Check sheet for the modelled part. Datum: model origin and axes. Units: mm. Face numbers are marked on the shaded views. A direction names the side the tool comes from. Round coordinates to 2 decimals unless told otherwise and drop trailing zeros. Order: outer loops, then holes, each group sorted by start corner. A loop starts at its lowest first (then second) coordinate and runs counter-clockwise, first axis right, second up. Notation, with made-up numbers: M 59,19 L 79,19 A21 cw 79,32 Z; hole C 53.5,-9.5 d4. An arc over 180 degrees is marked long. One line per item, written item: value. Start each with the question number.
(1) Cross-section at B-B, the plane y = -57.5. Enter the section's corners in (x, z), and give its area (3 significant figures).
(2) Cross-section at A-A, the plane x = -85. Enter the section's corners in (y, z).
(3) Access from +Z, -Z, +X, -X, +Y, -Y to the whole of each face (thin tool, end or side, straight path). Record for the marked faces 1 and 2.
(4) Thickness scan on L1, parallel to Z at x = -85, y = -61.7; L2, parallel to Z at x = -82.25, y = -58; L3, parallel to X at y = -64.5, z = -4. Record the ranges inside material, lowest first.
(5) Release check for a two-part mould opening along X. For the marked faces 3, 4, 5 and 6 record: released by +X, released by -X, zero draft, split by the parting line, or undercut.
(6) Cross-section at C-C, the plane y = -64.5. Enter the section's corners in (x, z).
(7) Depth check by flat-ended pin: pin 1 Ø3.5 at (x, z) = (-85.5, 8) entering from +Y; pin 2 Ø8 at (x, z) = (-85, 0) entering from -Y; pin 3 Ø1.6 at (x, z) = (-85, -19.25) entering from -Y. Enter the tip coordinate at first touch or a pass-through.
(8) Cross-section at D-D, the plane z = 8.25. Enter the section's corners in (x, y), and give its area (3 significant figures).
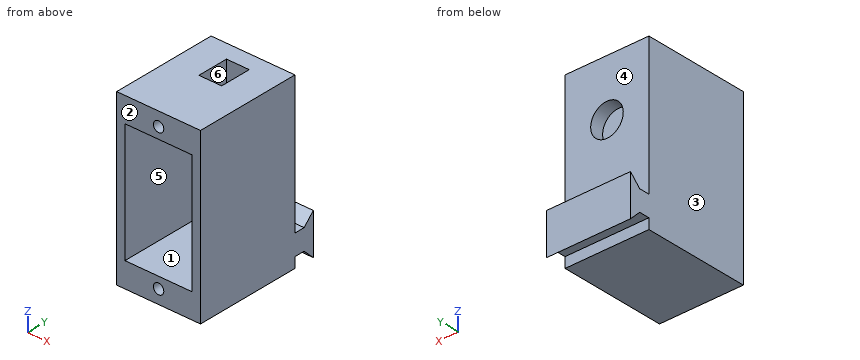
from build123d import *

# Parameters (mm, degrees)
BOSS_EXTRUDE1_START = -56.075
SKETCH1_W           = 16.2
SKETCH1_H           = 32.8
BOSS_EXTRUDE1_DEPTH = 10.275
BOSS_EXTRUDE2_START = -85
BOSS_EXTRUDE2_DEPTH = 8.1
CUT_EXTRUDE1_START  = -57.725
SKETCH3_W           = 13
SKETCH3_H           = 23.2
CUT_EXTRUDE1_DEPTH  = 8.625
CUT_EXTRUDE2_START  = -63.35
SKETCH4_R           = 1
CUT_EXTRUDE2_DEPTH  = 3
CUT_EXTRUDE3_START  = -63.35
SKETCH5_R           = 1
CUT_EXTRUDE3_DEPTH  = 3
CUT_EXTRUDE4_START  = -47.1
SKETCH6_R           = 3.15
CUT_EXTRUDE4_DEPTH  = 1.3
CUT_EXTRUDE5_START  = 8.5
SKETCH7_W           = 4.4
SKETCH7_H           = 6
CUT_EXTRUDE5_DEPTH  = 2.4


with BuildPart() as part:
    # Sketch1 → Boss-Extrude1 (new, symmetric)
    with BuildSketch(Plane(origin=(0, 0, 0), x_dir=(1, 0, 0), z_dir=(0, 1, 0)).offset(BOSS_EXTRUDE1_START)):
        with Locations((-85, 5.5)):
            Rectangle(SKETCH1_W, SKETCH1_H)
    extrude(amount=BOSS_EXTRUDE1_DEPTH, both=True)

    # Sketch2 → Boss-Extrude2 (add, symmetric)
    with BuildSketch(Plane(origin=(0, 0, 0), x_dir=(0, 0, -1), z_dir=(1, 0, 0)).offset(BOSS_EXTRUDE2_START)):
        Polygon((19.9, -46.3), (15.9, -46.3), (15.9, -43.8), (13.9, -41.8), (21.9, -41.8), (19.9, -43.8), align=None)
    extrude(amount=BOSS_EXTRUDE2_DEPTH, both=True)

    # Sketch3 → Cut-Extrude1 (cut, symmetric)
    with BuildSketch(Plane(origin=(0, 0, 0), x_dir=(1, 0, 0), z_dir=(0, 1, 0)).offset(CUT_EXTRUDE1_START)):
        with Locations((-85, 5.5)):
            Rectangle(SKETCH3_W, SKETCH3_H)
    extrude(amount=CUT_EXTRUDE1_DEPTH, both=True, mode=Mode.SUBTRACT)

    # Sketch4 → Cut-Extrude2 (cut, symmetric)
    with BuildSketch(Plane(origin=(0, 0, 0), x_dir=(1, 0, 0), z_dir=(0, 1, 0)).offset(CUT_EXTRUDE2_START)):
        with Locations(Location((-85, 19.25, 0), (0, 0, 270))):
            Circle(SKETCH4_R)
    extrude(amount=CUT_EXTRUDE2_DEPTH, both=True, mode=Mode.SUBTRACT)

    # Sketch5 → Cut-Extrude3 (cut, symmetric)
    with BuildSketch(Plane(origin=(0, 0, 0), x_dir=(1, 0, 0), z_dir=(0, 1, 0)).offset(CUT_EXTRUDE3_START)):
        with Locations(Location((-85, -8.25, 0), (0, 0, 270))):
            Circle(SKETCH5_R)
    extrude(amount=CUT_EXTRUDE3_DEPTH, both=True, mode=Mode.SUBTRACT)

    # Sketch6 → Cut-Extrude4 (cut, symmetric)
    with BuildSketch(Plane(origin=(0, 0, 0), x_dir=(1, 0, 0), z_dir=(0, 1, 0)).offset(CUT_EXTRUDE4_START)):
        with Locations(Location((-85, 0, 0), (0, 0, 270))):
            Circle(SKETCH6_R)
    extrude(amount=CUT_EXTRUDE4_DEPTH, both=True, mode=Mode.SUBTRACT)

    # Sketch7 → Cut-Extrude5 (cut, symmetric)
    with BuildSketch(Plane.XY.offset(CUT_EXTRUDE5_START)):
        with Locations((-85, -52.1)):
            Rectangle(SKETCH7_W, SKETCH7_H)
    extrude(amount=CUT_EXTRUDE5_DEPTH, both=True, mode=Mode.SUBTRACT)


solid = part.part
Values found:
1. outline: M -93.1,-21.9 L -76.9,-21.9 L -76.9,10.9 L -93.1,10.9 Z; hole M -91.5,-17.1 L -78.5,-17.1 L -78.5,6.1 L -91.5,6.1 Z
1. area: 230 mm^2
2. outline: M -66.35,-21.9 L -45.8,-21.9 L -45.8,-19.9 L -43.8,-19.9 L -41.8,-21.9 L -41.8,-13.9 L -43.8,-15.9 L -45.8,-15.9 L -45.8,-3.15 L -48.4,-3.15 L -48.4,3.15 L -45.8,3.15 L -45.8,10.9 L -49.1,10.9 L -49.1,-17.1 L -66.35,-17.1 L -66.35,-18.25 L -60.35,-18.25 L -60.35,-20.25 L -66.35,-20.25 Z; M -66.35,6.1 L -55.1,6.1 L -55.1,10.9 L -66.35,10.9 L -66.35,9.25 L -60.35,9.25 L -60.35,7.25 L -66.35,7.25 Z
3. face 1: -Y
3. face 2: +Z, -Z, +X, -X, -Y
4. L1: -21.9 to -20.25, -18.25 to -17.1, 6.1 to 7.25, 9.25 to 10.9
4. L2: -21.9 to -17.1, 6.1 to 10.9
4. L3: -93.1 to -91.5, -78.5 to -76.9
5. face 3: released by -X
5. face 4: zero draft
5. face 5: undercut
5. face 6: undercut
6. outline: M -93.1,-21.9 L -76.9,-21.9 L -76.9,10.9 L -93.1,10.9 Z; hole M -91.5,-17.1 L -78.5,-17.1 L -78.5,6.1 L -91.5,6.1 Z; hole C -85,-19.25 d2; hole C -85,8.25 d2
7. pin 1: y = -45.8
7. pin 2: y = -49.1
7. pin 3: y = -60.35
8. outline: M -93.1,-66.35 L -86,-66.35 L -86,-60.35 L -84,-60.35 L -84,-66.35 L -76.9,-66.35 L -76.9,-45.8 L -93.1,-45.8 Z; hole M -87.2,-55.1 L -82.8,-55.1 L -82.8,-49.1 L -87.2,-49.1 Z
8. area: 295 mm^2
